Answer from the drawing. Dimensions are ordinates in mm from the lowest x, y and z of the part. Give positions to 0.01 mm unless a question says otherwise; leave off trailing zeros. Write each loop counter-clockwise with the first axis right and the second up, starting at its lowest first coordinate (ties: lowest second). Pieces come first, ordered by that corner, then holes.
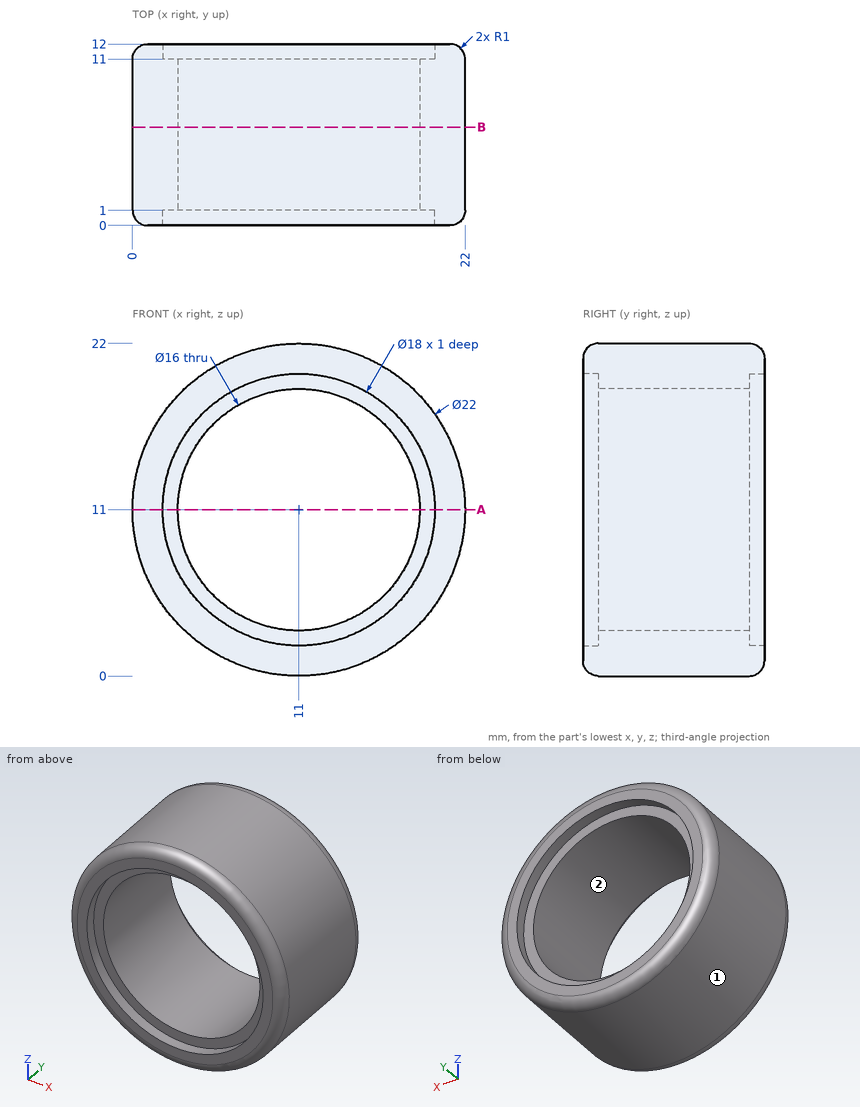
Item 1: Consider probe 1 along X at (y, z) = (5, 15.5); probe 2 along X at (y, z) = (11.45, 11); probe 3 along Z at (x, y) = (11.25, 6). Determine where each line is inside the solid, lowest interval first.
Conclusion:
probe 1: x = 0.96 to 4.39, 17.61 to 21.04
probe 2: x = 0.11 to 2, 20 to 21.89
probe 3: z = 0 to 3, 19 to 22
Item 2: A cutting plane is placed at B-B, the plane y = 6.5. Give the vertices of the cut face in (x, z), plus the area to 3 significant figures.
Conclusion:
outline: circle Ø22 at (11, 11); hole circle Ø16 at (11, 11)
area: 179 mm2
Item 3: Each of these flat-tipped pins is pushed along its axis until it touches: P1, Ø1, axis at x = 14.5, y = 3, coming from the -Z side; P2, Ø1.5, axis at x = 10, y = 6.5, coming from the -Z side; P3, Ø3, axis at x = 17.5, z = 13, coming from the -Y side; P4, Ø13, axis at x = 11, z = 11, coming from the +Y side. Where does it stop, or does it pass through?
Conclusion:
P1: stops at z = 0.42
P2: stops at z = 0
P3: stops at y = 1
P4: passes through
Item 4: Determine the mould class of the marked faces 1 and 2 for opening direction X: pulls with the +X half, pulls with the -X half, needs draft (parallel to the pull), parting line crosses it, or undercut.
Conclusion:
face 1: parting line crosses it
face 2: undercut
Item 5: A cutting plane is placed at A-A, the plane z = 11. Give the vertices of the cut face in (x, y).
Conclusion:
outline: (0, 1) arc R1 ccw to (1, 0) - (2, 0) - (2, 1) - (3, 1) - (3, 11) - (2, 11) - (2, 12) - (1, 12) arc R1 ccw to (0, 11) - close; (19, 1) - (20, 1) - (20, 0) - (21, 0) arc R1 ccw to (22, 1) - (22, 11) arc R1 ccw to (21, 12) - (20, 12) - (20, 11) - (19, 11) - close
